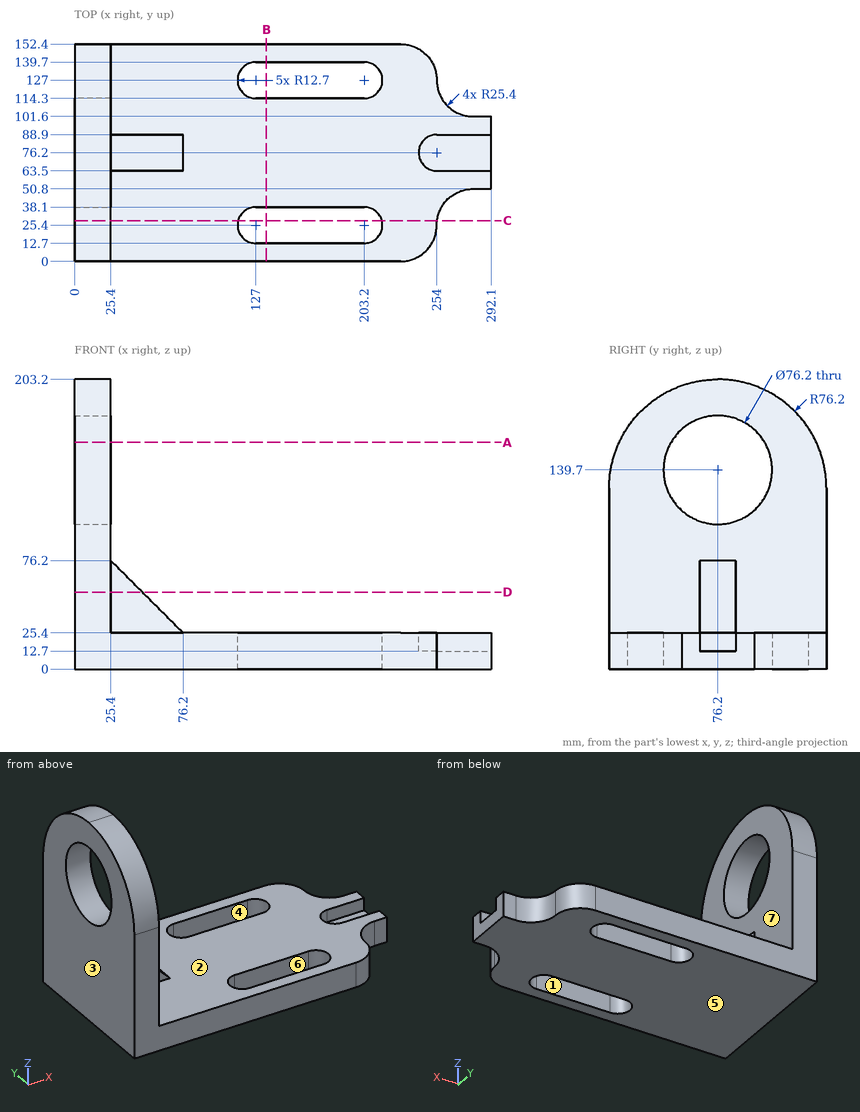
Can you work these out from the drawing? Everything is in mm from the part's minimum corner. A direction names the side the tool comes from. Coordinates: 2 decimals unless noted, no trailing zeros. Write each loop counter-clockwise with the first axis right and the second up, starting at its lowest first coordinate (ties: lowest second). Pieces come first, ordered by that corner, then holes. Notation, with made-up numbers: (-35, -7) -> (-25, -7) arc R23 ccw to (-25, 31) -> close; hole circle Ø4 at (-7, 75.5). An arc over 180 degrees is marked (long way). Write each question's results on one line, items separated by ' | '. Start each with the question number.
Item 1: If we section it at B-B, the plane x = 134.5: Write out the boundary of the cut face in (y, z).
Item 2: If we section it at A-A, the plane z = 159: Write out the boundary of the cut face in (x, y), and give its area (3 significant figures).
Item 3: Thinking about a two-plate mould opening in X: for the marked faces 4, 5, 6 and 7, which applies, released by +X, released by -X, zero draft, split by the parting line, or undercut?
Item 4: On a 3-axis mill with a long thin cutter (end or side, diameter ignored), from which of +Z, -Z, +X, -X, +Y, -Y can I reach the whole of each face in a straight line? I mean the marked faces 1, 2 and 3. Say none if no direction works.
Item 5: I'm going to push flat-ended pins straight in: P1, Ø1, axis at x = 81.5, y = 52, coming from the -Z side; P2, Ø15, axis at x = 42, z = 56.5, coming from the +Y side; P3, Ø10, axis at x = 286, z = 10, coming from the -Y side; P4, Ø8, axis at y = 99, z = 78, coming from the +X side. Where does each tip first touch, or does it pass through?
Item 6: If we section it at D-D, the plane z = 54: Write out the boundary of the cut face in (x, y).
Item 7: If we section it at C-C, the plane y = 28.5: Write out the boundary of the cut face in (x, z).
Item 8: Please list where these lines run through material, in increasing order: probe 1 along Z at (x, y) = (7, 76); probe 2 along Z at (x, y) = (57, 96).
Answer block:
1) outline: (0, 0) -> (12.7, 0) -> (12.7, 25.4) -> (0, 25.4) -> close; (38.1, 0) -> (114.3, 0) -> (114.3, 25.4) -> (38.1, 25.4) -> close; (139.7, 0) -> (152.4, 0) -> (152.4, 25.4) -> (139.7, 25.4) -> close
2) outline: (0, 7.04) -> (25.4, 7.04) -> (25.4, 43.35) -> (0, 43.35) -> close; (0, 109.05) -> (25.4, 109.05) -> (25.4, 145.36) -> (0, 145.36) -> close | area: 1,840 mm²
3) face 4: undercut | face 5: zero draft | face 6: undercut | face 7: released by +X
4) face 1: +Z, -Z | face 2: +Z, +X | face 3: +Z, -Z, -X, +Y, -Y
5) P1: z = 0 | P2: y = 88.9 | P3: y = 50.8 | P4: x = 25.4
6) outline: (0, 0) -> (25.4, 0) -> (25.4, 63.5) -> (47.6, 63.5) -> (47.6, 88.9) -> (25.4, 88.9) -> (25.4, 152.4) -> (0, 152.4) -> close
7) outline: (0, 0) -> (114.68, 0) -> (114.68, 25.4) -> (25.4, 25.4) -> (25.4, 186.42) -> (0, 186.42) -> close; (215.52, 0) -> (254.19, 0) -> (254.19, 25.4) -> (215.52, 25.4) -> close
8) probe 1: 0 to 101.6, 177.8 to 203.2 | probe 2: 0 to 25.4
